```python
from build123d import *

# Parameters (mm, degrees)
F2_W = 33.6
F2_H = 15.6
F4_R = 1


with BuildPart() as f1:
    # F0 (on Front) → F1 (revolve)
    with BuildSketch(Plane.XZ):
        with BuildLine():
            Line((3, 44.8), (3, 0))
            Line((3, 0), (25.6, 0))
            Line((25.6, 0), (25.6, 41))
            Line((25.6, 41), (20.6, 46))
            Line((20.6, 46), (7.75, 46))
            Line((7.75, 46), (6.9893398282, 45.2393398282))
            ThreePointArc((6.9893398282, 45.2393398282), (6.502704805, 44.9141807012), (5.9286796564, 44.8))
            Line((5.9286796564, 44.8), (3, 44.8))
        make_face()
    revolve(axis=Axis((0, 0, -6.1797830276), (0, 0, -1)))

    # F2 (on Front) → F3 (revolve, cut)
    with BuildSketch(Plane.XZ):
        with Locations((-8.8, 28.5)):
            Rectangle(F2_W, F2_H)
    revolve(axis=Axis((-34.5689574801, 0, 20.7), (-1, 0, 0)), mode=Mode.SUBTRACT)

    # F4
    f4_edges = [f1.edges().sort_by_distance(p)[0] for p in [
        (8, 0, 5.1),
    ]]
    fillet(f4_edges, radius=F4_R)

    # F5: F1 across plane


with BuildPart() as f1_1:
    add(f1.part)
    add(f1.part.mirror(Plane.XY))


solid = f1_1.part
```
Source: CAD feature listing. Evaluate the final solid. Frame: model axes, mm. A direction names the side the tool comes from. Round coordinates to 2 decimals unless told otherwise and drop trailing zeros. Loops run counter-clockwise (first coordinate to the right, second up) from the corner with the lowest first, then second, coordinate; pieces in that order, holes last. Notation, with made-up numbers: M -38.5,65 L -13.5,65 A24 ccw -13.5,98 Z; hole C 37,49 d11. An arc over 180 degrees is marked long. Use a Markdown table: item, result. Add a question column.
1. Contact query for flat-ended pins moving along their axis: P1, Ø6, axis at x = 4, y = -2, coming from the -Z side; P2, Ø3, axis at x = -9, z = -3, coming from the +Y side; P3, Ø6, axis at x = 0.5, y = -0.5, coming from the +Z side; P4, Ø5, axis at x = 0, y = 0, coming from the -Z side. Output: stop coordinate, or through.
2. Section query C-C on z = 20.7. Return the cut outline in (x, y).
3. Section query B-B on y = -1. Give the number of separate pieces and of enclosed holes in the cut face, then the cut area to 3 significant figures.
4. Mould query, pull axis X, two halves, no side actions, for faces 3 (the flat face through (8, 0, 21)), 4 (the conical face through (-4.518, 20.347, 45.757)), 5 (the flat face through (-3, -1, -44.8)), 6 (the flat face through (-3, -1, 44.8)). Classes: pulls with the +X half, pulls with the -X half, needs draft (parallel to the pull), parting line crosses it, or undercut.
5. Reachability of faces 1 (the flat face through (8, 0, -21)), 2 (the cylindrical face through (-3, 0, 40)) from +Z, -Z, +X, -X, +Y, -Y: full face, straight path, thin tool, end or side. Return the list, or none.
6. Line query: line 1 (Z direction, x = -4, y = 0); line 2 (Z direction, x = -5, y = 3); line 3 (X direction, y = 0, z = 1.8). Output: solid intervals per line, ascending.
Reported:
| question | item | result |
|---|---|---|
| 1 | P1 | stops at z = -45.72 |
| 1 | P2 | stops at y = 24.48 |
| 1 | P3 | stops at z = 44.8 |
| 1 | P4 | passes through |
| 2 | outline | M -20.3,-15.6 A25.6 ccw long -20.3,15.6 L 7,15.6 A1 cw 8,14.6 L 8,-14.6 A1 cw 7,-15.6 Z |
| 3 | separate pieces | 4 |
| 3 | enclosed holes | 0 |
| 3 | area | 2,380 mm² |
| 4 | face 3 | pulls with the -X half |
| 4 | face 4 | parting line crosses it |
| 4 | face 5 | undercut |
| 4 | face 6 | undercut |
| 5 | face 1 | -X |
| 5 | face 2 | +Z, -Z |
| 6 | line 1 | z = -44.8 to -36.3, -5.1 to 5.1, 36.3 to 44.8 |
| 6 | line 2 | z = -44.8 to -36.01, -5.39 to 5.39, 36.01 to 44.8 |
| 6 | line 3 | x = -25.6 to -3, 3 to 25.6 |
